Input: dimensioned drawing with shaded views. Units: mm. Origin: part minimum x, y, z. Give positions to 0.01 mm unless a question says otherwise; leave off trailing zeros. Loops run counter-clockwise (first coordinate to the right, second up) from the corner with the lowest first, then second, coordinate; pieces in that order, holes last.
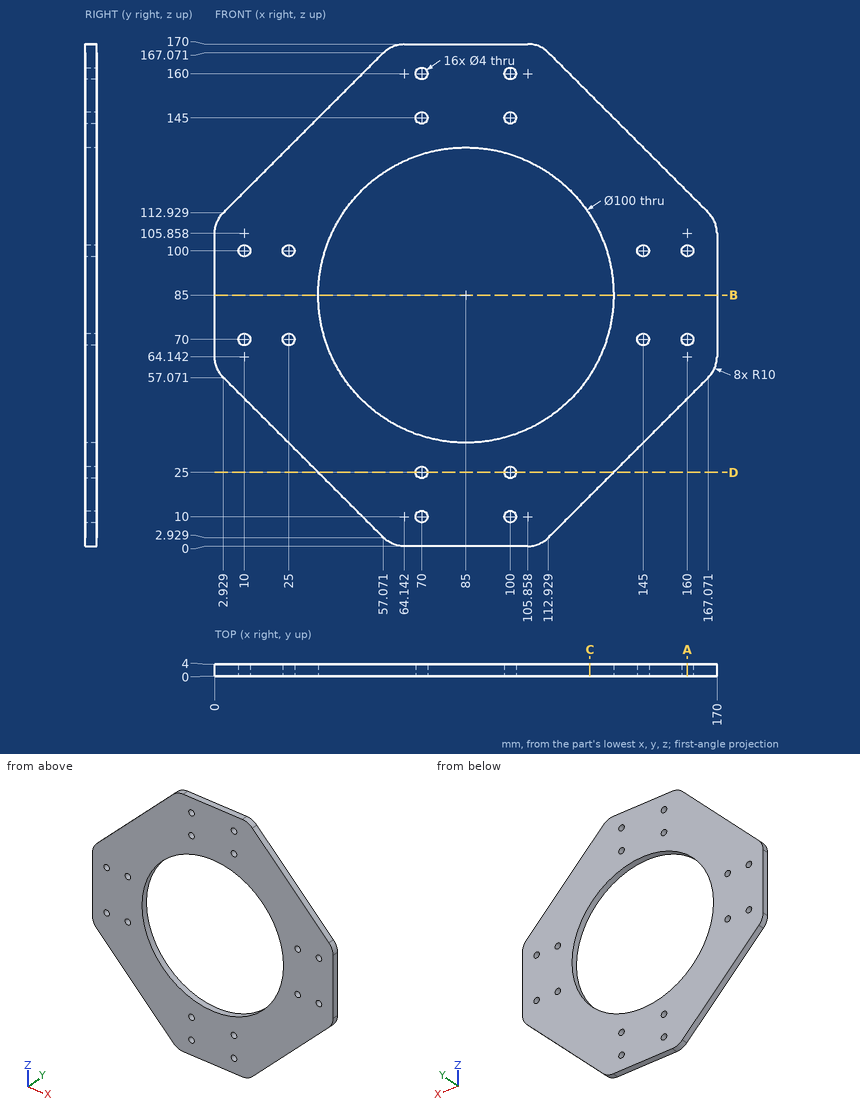
(1) Section B-B, the plane z = 85. Return the cut outline in (x, y), then the cut area to 3 significant figures.
A:
outline: (0, 0) - (35, 0) - (35, 4) - (0, 4) - close; (135, 0) - (170, 0) - (170, 4) - (135, 4) - close
area: 280 mm2
(2) Section C-C, the plane x = 127. Return the cut outline in (y, z), then the cut area to 3 significant figures.
A:
outline: (0, 17) - (4, 17) - (4, 57.87) - (0, 57.87) - close; (0, 112.13) - (4, 112.13) - (4, 153) - (0, 153) - close
area: 327 mm2
(3) Section A-A, the plane x = 160. Return the cut outline in (y, z), then the cut area to 3 significant figures.
A:
outline: (0, 50) - (4, 50) - (4, 68) - (0, 68) - close; (0, 72) - (4, 72) - (4, 98) - (0, 98) - close; (0, 102) - (4, 102) - (4, 120) - (0, 120) - close
area: 248 mm2
(4) First-contact query: pin 1 (4.5 mm diameter, centred on x = 160, z = 100, fed in from +Y); pin 2 (1.5 mm diameter, centred on x = 126.5, y = 0.5, fed in from -Z); pin 3 (1.5 mm diameter, centred on x = 40, y = 3, fed in from +Z). Flat tips, straight axial feed; report the tip coordinate or a pass-through.
A:
pin 1: stops at y = 4
pin 2: stops at z = 15.75
pin 3: stops at z = 150.75
(5) Section D-D, the plane z = 25. Return the cut outline in (x, y).
A:
outline: (35, 0) - (68, 0) - (68, 4) - (35, 4) - close; (72, 0) - (98, 0) - (98, 4) - (72, 4) - close; (102, 0) - (135, 0) - (135, 4) - (102, 4) - close
(6) Ray query, line 1 along X through (y, z) = (2.6, 145); line 2 along X through (y, z) = (1.85, 70); line 3 along X through (y, z) = (1.8, 160). Return the intervals inside material, ascending.
A:
line 1: x = 35 to 68, 72 to 98, 102 to 135
line 2: x = 0 to 8, 12 to 23, 27 to 37.3, 132.7 to 143, 147 to 158, 162 to 170
line 3: x = 50 to 68, 72 to 98, 102 to 120
